Work out the finished part from the listing and answer in its coordinate system (mm). Round coordinates to 2 decimals unless told otherwise and drop trailing zeros. Order: outer loops, then holes, each group sorted by start corner. A loop starts at its lowest first (then second) coordinate and runs counter-clockwise, first axis right, second up. Notation, with made-up numbers: (60.25, 42) -> (69.25, 42) arc R24 ccw to (69.25, 81) -> close; hole circle Ø11 at (-16, 45.25). An arc over 180 degrees is marked (long way). Use one line per item in the form item = value.
Autodesk Inventor part; units mm, degrees
ref_plane "YZ Plane" through (0, 0, 0) normal (1, 0, 0) x (0, 1, 0)
ref_plane "XZ Plane" through (0, 0, 0) normal (0, 1, 0) x (-1, 0, 0)
ref_plane "XY Plane" through (0, 0, 0) normal (0, 0, 1) x (1, 0, 0)
sketch "Sketch1" plane through (0, 0, 0) normal (0, 0, 1) x (1, 0, 0)
  line L0 (-76, 61) -> (76, 61)
  line L1 (76, 61) -> (76, -61)
  line L2 (76, -61) -> (-76, -61)
  line L3 (-76, -61) -> (-76, 61)
  line L4 (-69.5, 55) -> (69.5, 55)
  line L5 (69.5, 55) -> (69.5, -55)
  line L6 (69.5, -55) -> (-69.5, -55)
  line L7 (-69.5, -55) -> (-69.5, 55)
  line L8 (84, 69) -> (-84, 69)
  line L9 (-84, 69) -> (-84, -69)
  line L10 (-84, -69) -> (84, -69)
  line L11 (84, -69) -> (84, 69)
  line L12 (72.5, 58) -> (-72.5, 58)
  line L13 (-72.5, 58) -> (-72.5, -58)
  line L14 (-72.5, -58) -> (72.5, -58)
  line L15 (72.5, -58) -> (72.5, 58)
  line L16 (0, 109.6961) -> (0, -131.8013)
  line L17 (-145.0248, 0) -> (154.2595, 0)
  line L18 (77, -62) -> (77, 62)
  line L19 (77, 62) -> (-77, 62)
  line L20 (-77, 62) -> (-77, -62)
  line L21 (-77, -62) -> (77, -62)
  point P0 (0, 0)
  point P1 (-68, -65)
  point P2 (-80, -53)
  point P3 (-22.6667, -65)
  point P4 (22.6667, -65)
  point P5 (68, -65)
  point P6 (-80, 0)
  point P7 (-80, 53)
  point P8 (80, -53)
  point P9 (80, 0)
  point P10 (80, 53)
  point P11 (-68, 65)
  point P12 (-22.6667, 65)
  point P13 (22.6667, 65)
  point P14 (68, 65)
  dimension "d0" = 152
  dimension "d1" = 122
  dimension "d2" = 139
  dimension "d3" = 110
  dimension "d4" = 6
  dimension "d5" = 6.5
  dimension "d6" = 8
  dimension "d7" = 3
  dimension "d44" = 69.5
  dimension "d45" = 55
  dimension "d84" = 4
  dimension "d85" = 4
  dimension "d87" = 16
  dimension "d88" = 16
  dimension "d89" = 168
  dimension "d90" = 138
  dimension "d93" = 45.3333
  dimension "d100" = 53
  dimension "d119" = 1
extrude "Extrusion1" add sketch "Sketch1" along normal blind 3.2 contours L19 L20 L17 L9 L8 L16 | L16 L8 L11 L17 L18 L19 | L20 L21 L16 L10 L9 L17 | L17 L11 L10 L16 L21 L18
fillet "Fillet8" radius 10 4 edges at (-84, -69, 1.6) (84, -69, 1.6) (84, 69, 1.6) (-84, 69, 1.6)
hole "Hole2" at (-68, -65, 0) at (-80, -53, 0) at (-22.6667, -65, 0) at (22.6667, -65, 0) at (68, -65, 0) at (-80, 0, 0) at (-80, 53, 0) at (80, 53, 0) at (80, 0, 0) at (80, -53, 0) at (-68, 65, 0) at (-22.6667, 65, 0) at (22.6667, 65, 0) at (68, 65, 0) direction (0, 0, 1) diameter 3.2 depth 3.2
fillet "Fillet9" radius 3 4 edges at (77, 62, 1.6) (-77, 62, 1.6) (-77, -62, 1.6) (77, -62, 1.6)
equation "\"d4\" = -0.5 * d3 + 0.5 * d1"
equation "\"d5\" = -0.5 * d2 + 0.5 * d0"
properties part number "3DP_PLA_Front_filter_mount_hood_spacer"
Item 1: The part is cut by section B-B, the plane x = -56. Give the vertices of the cut face in (y, z).
Findings:
outline = (-69, 0) -> (-62, 0) -> (-62, 3.2) -> (-69, 3.2) -> close; (62, 0) -> (69, 0) -> (69, 3.2) -> (62, 3.2) -> close
Item 2: Flat-ended cylindrical pins translate along their axes: P1, Ø2.5, axis at x = -68, y = -65, coming from the -Z side; P2, Ø5, axis at x = -22.67, y = 65, coming from the +Z side. Find the tip coordinate at first contact, or state that the pin passes through.
Findings:
P1 = through
P2 = 3.2
Item 3: Consider line 1 along X through (y, z) = (-53, 2.05); line 2 along Y through (x, z) = (68, 0.9); line 3 along Y through (x, z) = (4, 3). Determine where each line is inside the solid, lowest interval first.
Findings:
line_1 = -84 to -81.6, -78.4 to -77, 77 to 78.4, 81.6 to 84
line_2 = -69 to -66.6, -63.4 to -62, 62 to 63.4, 66.6 to 69
line_3 = -69 to -62, 62 to 69
Item 4: The part is cut by section C-C, the plane z = 0.6. Give the number of separate pieces and of enclosed holes in the cut face, and give its area (3 significant figures).
Findings:
separate_pieces = 1
enclosed_holes = 15
area = 3,900 mm^2
Item 5: The part is cut by section A-A, the plane y = 13. Give the vertices of the cut face in (x, z).
Findings:
outline = (-84, 0) -> (-77, 0) -> (-77, 3.2) -> (-84, 3.2) -> close; (77, 0) -> (84, 0) -> (84, 3.2) -> (77, 3.2) -> close
